Can you work these out from the drawing? Everything is in mm from the part's minimum corner. Coordinates: 2 decimals unless noted, no trailing zeros. Loops run counter-clockwise (first coordinate to the right, second up) from the corner with the lowest first, then second, coordinate; pieces in that order, holes last. Notation, with made-up numbers: (-8, 81) - (47, 81) arc R27 cw to (47, 112) - close; hole circle Ø3 at (13.5, -10). An arc over 180 degrees is marked (long way). Put each result on its own line as item: value. Start each with the question number.
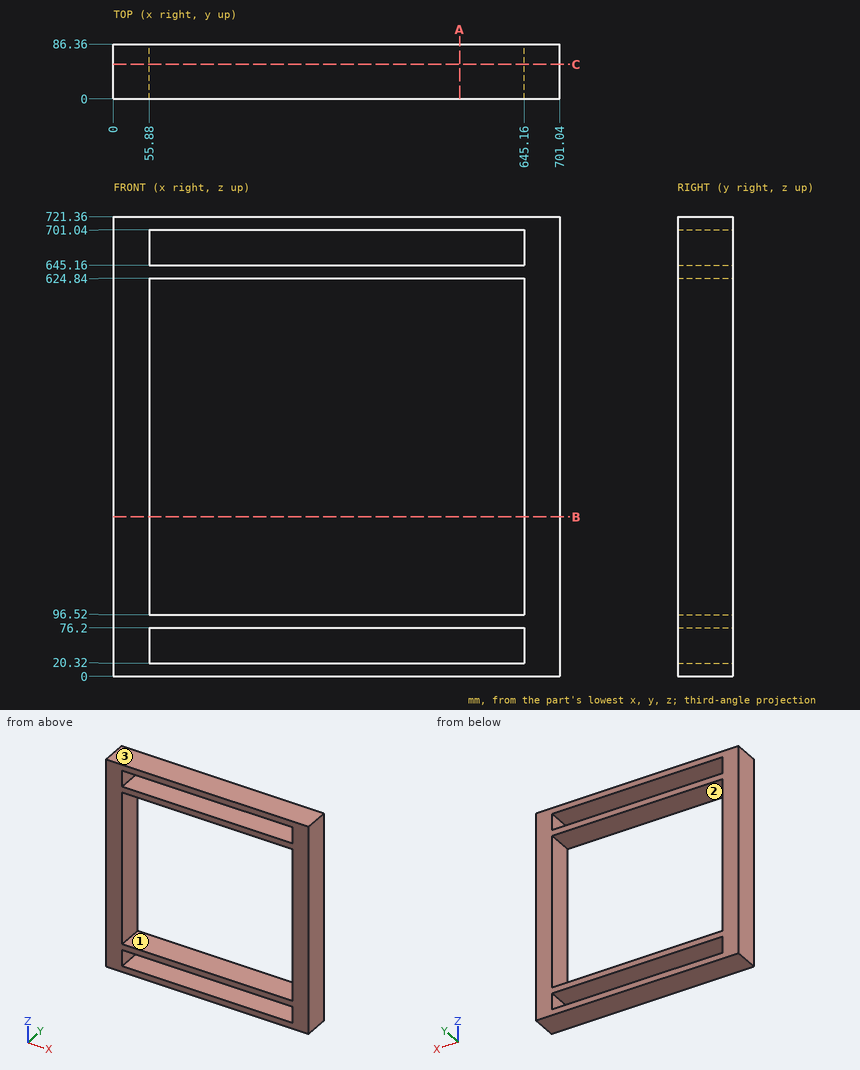
(1) I want a section at A-A on x = 544. List the corners of the cut face in (y, z) for me, and give its area (3 significant figures).
(2) If we mould it in two halves opening along X, with no side actions, what happens to the marked faces 1, 2 and 3? For each: pulls with the +X half, pulls with the -X half, needs draft (parallel to the pull), parting line crosses it, or undercut.
(3) For pin 1 Ø1.5 at (y, z) = (49, 85.5) entering from -X, with a flat end and sliding along its axis, tell me the tip position at first contact or that it passes through.
(4) I need wall thicknesses on L1, parallel to Z at x = 336, y = 77; L2, parallel to X at y = 20, z = 230. Which ranges of each line are inside material? Lowest first, please. Write a range as [from, to].
(5) I want a section at B-B on z = 250. List the corners of the cut face in (x, y) for me, and give its area (3 significant figures).
(6) I want a section at C-C on y = 54.5. List the corners of the cut face in (x, z) for me.
Answer sheet:
1. outline: (0, 0) - (86.36, 0) - (86.36, 20.32) - (0, 20.32) - close; (0, 76.2) - (86.36, 76.2) - (86.36, 96.52) - (0, 96.52) - close; (0, 624.84) - (86.36, 624.84) - (86.36, 645.16) - (0, 645.16) - close; (0, 701.04) - (86.36, 701.04) - (86.36, 721.36) - (0, 721.36) - close
1. area: 7,020 mm^2
2. face 1: undercut
2. face 2: undercut
2. face 3: needs draft
3. pin 1: stops at x = 0
4. L1: z = [0, 20.32], [76.2, 96.52], [624.84, 645.16], [701.04, 721.36]
4. L2: x = [0, 55.88], [645.16, 701.04]
5. outline: (0, 0) - (55.88, 0) - (55.88, 86.36) - (0, 86.36) - close; (645.16, 0) - (701.04, 0) - (701.04, 86.36) - (645.16, 86.36) - close
5. area: 9,650 mm^2
6. outline: (0, 0) - (701.04, 0) - (701.04, 721.36) - (0, 721.36) - close; hole (55.88, 20.32) - (645.16, 20.32) - (645.16, 76.2) - (55.88, 76.2) - close; hole (55.88, 96.52) - (645.16, 96.52) - (645.16, 624.84) - (55.88, 624.84) - close; hole (55.88, 645.16) - (645.16, 645.16) - (645.16, 701.04) - (55.88, 701.04) - close
